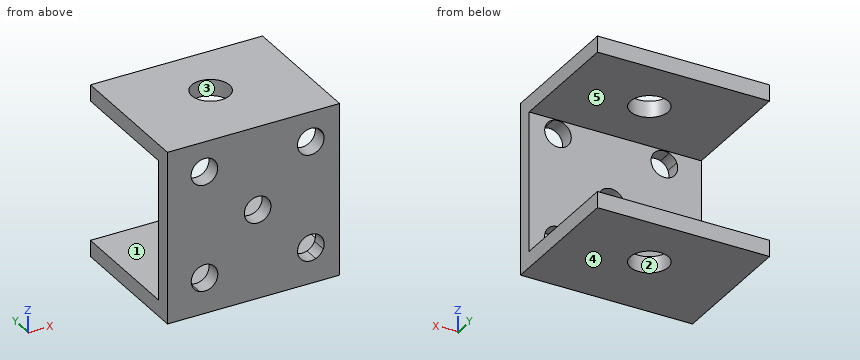
Autodesk Inventor part; units mm, degrees
ref_plane "YZ Plane" through (0, 0, 0) normal (1, 0, 0) x (0, 1, 0)
ref_plane "XZ Plane" through (0, 0, 0) normal (0, 1, 0) x (-1, 0, 0)
ref_plane "XY Plane" through (0, 0, 0) normal (0, 0, 1) x (1, 0, 0)
sketch "Sketch1" plane through (0, 0, 0) normal (0, 1, 0) x (-1, 0, 0)
  line L0 (16.1798, 16.1798) -> (0, 16.1798)
  line L1 (0, 16.1798) -> (0, 0)
  line L2 (0, 0) -> (16.1798, 0)
  line L3 (16.1798, 0) -> (16.1798, 16.1798)
  dimension "d0" = 16.1798
  dimension "d1" = 16.1798
extrude "Extrusion1" add sketch "Sketch1" along normal blind 1.4478
sketch "Sketch2" plane through (0, 1.4478, 0) normal (0, 1, 0) x (1, 0, 0)
  line L0 (0, -16.1798) -> (0, 0)
  line L1 (-16.1798, 0) -> (-16.1798, -16.1798)
  line L2 (0, 0) -> (-16.1798, 0)
  line L3 (-16.1798, 0) -> (-16.1798, -1.524)
  line L4 (-16.1798, -1.524) -> (0, -1.524)
  line L5 (0, -1.524) -> (0, 0)
  line L6 (-16.1798, -16.1798) -> (0, -16.1798)
  line L7 (0, -16.1798) -> (0, -14.6558)
  line L8 (0, -14.6558) -> (-16.1798, -14.6558)
  line L9 (-16.1798, -14.6558) -> (-16.1798, -16.1798)
  dimension "d4" = 1.524
  dimension "d5" = 1.524
extrude "Extrusion2" add sketch "Sketch2" along normal blind 11.2776 contours L6 L1 L8 L0 | L4 L1 L2 L0
sketch "Sketch3" plane through (-16.1798, 0, 16.1798) normal (0, 0, 1) x (1, 0, 0)
  circle A0 centre (8.0899, 7.0866) radius 1.7859
  line L0 (0, 1.4478) -> (0, 12.7254) construction
  line L1 (0, 7.0866) -> (16.1798, 7.0866) construction
  line L2 (16.1798, 1.4478) -> (16.1798, 12.7254) construction
  line L3 (16.1798, 12.7254) -> (0, 12.7254) construction
  line L4 (8.0899, 12.7254) -> (8.0899, 0) construction
  line L5 (0, 0) -> (16.1798, 0) construction
  dimension "d8" = 3.5719
extrude "Extrusion3" cut sketch "Sketch3" against normal through all
sketch "Sketch4" plane through (0, 1.4478, 0) normal (0, 1, 0) x (1, 0, 0)
  circle A0 centre (-7.7025, -8.3571) radius 1.25
  arc A1 (-13.8611, -2.8949) -> (-13.1534, -2.1884) centre (-12.6979, -3.3525) ccw
  arc A2 (-2.2403, -2.1985) -> (-1.5338, -2.9063) centre (-2.6979, -3.3617) ccw
  arc A3 (-1.5439, -13.8193) -> (-2.2517, -14.5258) centre (-2.7072, -13.3617) ccw
  arc A4 (-13.1648, -14.5157) -> (-13.8712, -13.8079) centre (-12.7072, -13.3525) ccw
  circle A5 centre (-12.7072, -13.3525) radius 1.25
  circle A6 centre (-12.6979, -3.3525) radius 1.25
  circle A7 centre (-12.6979, -3.3525) radius 1.25
  circle A8 centre (-2.7072, -13.3617) radius 1.25
  circle A9 centre (-2.6979, -3.3617) radius 1.25
  point P0 (0, 0)
extrude "Extrusion4" cut sketch "Sketch4" against normal through all
properties part number "channel1 of lift pivot"
Here's how the part is built. I have some questions about the finished solid (model axes, mm). Face numbers are marked on the shaded views. A direction names the side the tool comes from. Coordinates: 2 decimals unless noted, no trailing zeros. Loops run counter-clockwise (first coordinate to the right, second up) from the corner with the lowest first, then second, coordinate; pieces in that order, holes last.
1. Imagine slicing it at D-D, the plane z = 12.75. Please give me the cut outline in (x, y), and give its area (3 significant figures).
2. For P1, Ø3, axis at x = -8.09, y = 7.09, coming from the +Z side; P2, Ø4, axis at x = -11.5, z = 11, coming from the +Y side, each with a flat end and sliding along its axis, tell me the tip position at first contact or that it passes through.
3. Imagine slicing it at B-B, the plane y = 9.25. Please give me the cut outline in (x, z).
4. Imagine slicing it at A-A, the plane x = -12.75. Please give me the cut outline in (y, z), and give its area (3 significant figures).
5. For the marked faces 1 and 2, which set-ups out of +Z, -Z, +X, -X, +Y, -Y let a thin tool reach every point of the face, with its end or its side?
6. If we mould it in two halves opening along Z, with no side actions, what happens to the marked faces 3, 4 and 5? For each: pulls with the +Z half, pulls with the -Z half, needs draft (parallel to the pull), parting line crosses it, or undercut.
7. I need wall thicknesses on L1, parallel to Z at x = -7.75, y = 5.25; L2, parallel to Y at x = -7, z = 4.5; L3, parallel to X at y = 0.75, z = 8. Which ranges of each line are inside material? Lowest first, please.
8. Imagine slicing it at C-C, the plane z = 7.5. Please give me the cut outline in (x, y).
Taken from the geometry:
1. outline: (-16.18, 0) - (-13.8, 0) - (-13.8, 1.45) - (-16.18, 1.45) - close; (-11.61, 0) - (-3.8, 0) - (-3.8, 1.45) - (-11.61, 1.45) - close; (-1.62, 0) - (0, 0) - (0, 1.45) - (-1.62, 1.45) - close
1. area: 17.1 mm2
2. P1: passes through
2. P2: stops at y = 1.45
3. outline: (-16.18, 0) - (0, 0) - (0, 1.52) - (-16.18, 1.52) - close; (-16.18, 14.66) - (0, 14.66) - (0, 16.18) - (-16.18, 16.18) - close
4. outline: (0, 0) - (12.73, 0) - (12.73, 1.52) - (1.45, 1.52) - (1.45, 2.1) - (0, 2.1) - close; (0, 4.6) - (1.45, 4.6) - (1.45, 12.1) - (0, 12.1) - close; (0, 14.6) - (1.45, 14.6) - (1.45, 14.66) - (12.73, 14.66) - (12.73, 16.18) - (0, 16.18) - close
4. area: 50.6 mm2
5. face 1: +X, -X, +Y
5. face 2: +Z, -Z
6. face 3: needs draft
6. face 4: pulls with the -Z half
6. face 5: undercut
7. L1: z = 0 to 1.52, 14.66 to 16.18
7. L2: y = 0 to 1.45
7. L3: x = -16.18 to -8.9, -6.5 to 0
8. outline: (-16.18, 0) - (-8.61, 0) - (-8.61, 1.45) - (-16.18, 1.45) - close; (-6.79, 0) - (0, 0) - (0, 1.45) - (-6.79, 1.45) - close
